Part model, mm, in its own coordinate system. Face numbers are marked on the shaded views. A direction names the side the tool comes from. Round coordinates to 2 decimals unless told otherwise and drop trailing zeros. Write each loop counter-clockwise with the first axis right and the second up, starting at its lowest first coordinate (ties: lowest second). Pieces come first, ordered by that corner, then holes. Notation, with made-up numbers: (68, 0.5) -> (84, 0.5) arc R18 ccw to (84, 12.5) -> close; hole circle Ø4 at (72, -34). An arc over 180 degrees is marked (long way). Use CSV: the item, a comma, the result in double quotes. Start each with the question number.
(1) Saw through at D-D (y = -101.5). Give the cut face in (x, z).
(2) Two-plate mould, pull along Y, no slides. Class the marked faces 1, 2 and 3: released by +Y, released by -Y, zero draft, split by the parting line, or undercut.
(3) Saw through at B-B (x = 0). Give the cut face in (y, z), plus the area to 3 significant figures.
(4) Drop flat-ended pins along their axis: pin 1 (11.5 mm diameter, centred on x = -28.73, z = 27.52, fed in from +Y); pin 2 (1.5 mm diameter, centred on y = -73, z = -5, fed in from -X); pin 3 (5 mm diameter, centred on y = -44, z = -21, fed in from -X); pin 4 (8 mm diameter, centred on x = 2, y = -47, fed in from +Z). Give the stop position or say it passes through.
(5) Saw through at A-A (z = 0). Give the cut face in (x, y), plus the area to 3 significant figures.
(6) Which spindle directions (+Z, -Z, +X, -X, +Y, -Y) get a long thin tool onto all of the face, cutting with end or side? Do the marked faces 4 and 5. Say none if no direction does.
(7) Saw through at C-C (y = -52.5). Give the cut face in (x, z), plus the area to 3 significant figures.
(8) Probe line 1 (Z direction, x = 28.5, y = -100.5); line 2 (Y direction, x = -28.5, z = -21.5); line 3 (Z direction, x = 0, y = -67). List the from-to ranges inside material, lowest first. Write a range as [from, to].
```python
from build123d import *

# Parameters (mm, degrees)
F0_W      = 76.2
F0_H      = 76.2
F1_DEPTH  = 19.05
F2_R      = 25.4
F3_DEPTH  = 76.2
F4_W      = 76.2
F4_H      = 76.2
F5_DEPTH  = 19.05
F6_R      = 19.05
F8_DEPTH  = 114.3
F9_R      = 6.35
F10_DEPTH = 114.3


with BuildPart() as f1:
    # F0 (on Front) → F1 (new body)
    with BuildSketch(Plane.XZ):
        Rectangle(F0_W, F0_H)
    extrude(amount=F1_DEPTH)

    # F2 (on face) → F3 (join)
    with BuildSketch(Plane.XZ.offset(19.05)):
        Circle(F2_R)
    extrude(amount=F3_DEPTH)

    # F4 (on face) → F5 (join)
    with BuildSketch(Plane.XZ.offset(95.25)):
        Rectangle(F4_W, F4_H)
    extrude(amount=F5_DEPTH)

    # F6 (on face) → F8 (cut)
    with BuildSketch(Plane.XZ.offset(114.3)):
        Circle(F6_R)
    extrude(amount=-F8_DEPTH, mode=Mode.SUBTRACT)

    # F9 (on face) → F10 (cut)
    with BuildSketch(Plane.XZ.offset(114.3)):
        with Locations((-28.725395, 27.522238)):
            Circle(F9_R)
        with Locations((-28.424606, -29.326973)):
            Circle(F9_R)
        with Locations((28.725393, -29.326973)):
            Circle(F9_R)
        with Locations((28.424604, 27.522238)):
            Circle(F9_R)
    extrude(amount=-F10_DEPTH, mode=Mode.SUBTRACT)


solid = f1.part
```
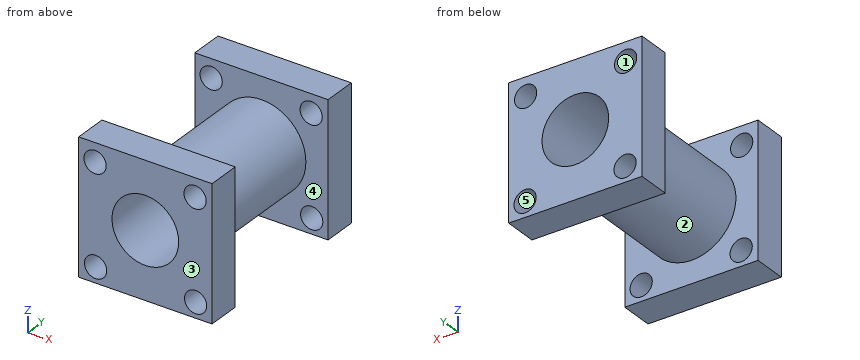
Answers:
1,outline,"(-38.1, -38.1) -> (38.1, -38.1) -> (38.1, 38.1) -> (-38.1, 38.1) -> close; hole circle Ø12.7 at (-28.73, 27.52); hole circle Ø12.7 at (-28.42, -29.33); hole circle Ø38.1 at (0, 0); hole circle Ø12.7 at (28.42, 27.52); hole circle Ø12.7 at (28.73, -29.33)"
2,face 1,"zero draft"
2,face 2,"undercut"
2,face 3,"released by -Y"
3,outline,"(-114.3, -38.1) -> (-95.25, -38.1) -> (-95.25, -25.4) -> (-19.05, -25.4) -> (-19.05, -38.1) -> (0, -38.1) -> (0, -19.05) -> (-114.3, -19.05) -> close; (-114.3, 19.05) -> (0, 19.05) -> (0, 38.1) -> (-19.05, 38.1) -> (-19.05, 25.4) -> (-95.25, 25.4) -> (-95.25, 38.1) -> (-114.3, 38.1) -> close"
3,area,"2,420 mm²"
4,pin 1,"passes through"
4,pin 2,"stops at x = -25.04"
4,pin 3,"stops at x = -17.4"
4,pin 4,"stops at z = 25.4"
5,outline,"(-38.1, -114.3) -> (-19.05, -114.3) -> (-19.05, 0) -> (-38.1, 0) -> (-38.1, -19.05) -> (-25.4, -19.05) -> (-25.4, -95.25) -> (-38.1, -95.25) -> close; (19.05, -114.3) -> (38.1, -114.3) -> (38.1, -95.25) -> (25.4, -95.25) -> (25.4, -19.05) -> (38.1, -19.05) -> (38.1, 0) -> (19.05, 0) -> close"
5,area,"2,420 mm²"
6,face 4,"none"
6,face 5,"+Y, -Y"
7,outline,"circle Ø50.8 at (0, 0); hole circle Ø38.1 at (0, 0)"
7,area,"887 mm²"
8,line 1,"z = [-38.1, -35.67], [-22.98, 21.17], [33.87, 38.1]"
8,line 2,"y = [-114.3, -95.25], [-19.05, 0]"
8,line 3,"z = [-25.4, -19.05], [19.05, 25.4]"
